```python
from build123d import *

# Parameters (mm, degrees)
SKETCH1_R           = 2.0701
BOSS_EXTRUDE1_DEPTH = 1.1684


with BuildPart() as part:
    # Sketch1 → Boss-Extrude1 (new body)
    with BuildSketch(Plane(origin=(0, 1.1684, 0), x_dir=(1, 0, 0), z_dir=(0, 1, 0))):
        with BuildLine():
            Line((16.856899662, 38.114124823), (13.80361258, 38.114124823))
            Line((13.80361258, 38.114124823), (-5.52378647, 18.786725773))
            Line((-5.52378647, 18.786725773), (-6.35, 16.792069862))
            Line((-6.35, 16.792069862), (-6.35, -10.541))
            Line((-6.35, -10.541), (-4.191, -12.7))
            Line((-4.191, -12.7), (4.191, -12.7))
            Line((4.191, -12.7), (6.35, -10.541))
            Line((6.35, -10.541), (6.35, 11.384871939))
            ThreePointArc((6.35, 11.384871939), (6.591682484, 12.599891837), (7.27993597, 13.62993597))
            Line((7.27993597, 13.62993597), (22.783868702, 29.133868702))
            Line((22.783868702, 29.133868702), (22.783868702, 32.187155783))
            Line((22.783868702, 32.187155783), (16.856899662, 38.114124823))
        make_face()
        with Locations((15.330256121, 30.660512242)):
            Circle(SKETCH1_R, mode=Mode.SUBTRACT)
        with Locations((0, 6.35)):
            Circle(SKETCH1_R, mode=Mode.SUBTRACT)
        with Locations((-2.085466914, 16.194084801)):
            Circle(SKETCH1_R, mode=Mode.SUBTRACT)
        with Locations((0, -6.35)):
            Circle(SKETCH1_R, mode=Mode.SUBTRACT)
        with Locations((6.35, 21.680256121)):
            Circle(SKETCH1_R, mode=Mode.SUBTRACT)
    extrude(amount=-BOSS_EXTRUDE1_DEPTH)


solid = part.part
```
Input: part model. Units: mm. Frame: model coordinates. A direction names the side the tool comes from. Coordinates: 2 decimals unless noted, no trailing zeros. Loops run counter-clockwise (first coordinate to the right, second up) from the corner with the lowest first, then second, coordinate; pieces in that order, holes last. Notation, with made-up numbers: M 14,-37 L 60,-37 A21 ccw 60,-10 Z; hole C 37.5,18 d4. An arc over 180 degrees is marked long. Use a Markdown table: item, result. Add a question column.
1) Draft query along X for faces 1 (the cylindrical face through (16.285, 0.592, -28.824)), 2 (the flat face through (5, 1.168, -13)), 3 (the flat face through (14.92, 0.59, -21.27)), 4 (the cylindrical face through (-0.97, 0.59, -17.94)). Return one class per face: +X half, -X half, draft (parallel to the pull), parting line (faces both ways), or undercut.
2) Section A-A, the plane z = 6.35. Return the cut outline in (x, y), plus the area to 3 significant figures.
3) Line query: L1, parallel to Z at x = 0.25, y = 0.65; L2, parallel to X at y = 0.8, z = -8.5; L3, parallel to Z at x = -1.75, y = 1. Output: solid intervals per line, ascending. Write a range as from..to.
4) Section C-C, the plane y = 0.25. Return the cut outline in (x, z) (3 decimals), plus the area to 3 significant figures.
5) Section D-D, the plane z = -24.5. Return the cut outline in (x, y), plus the area to 3 significant figures.
6) Section B-B, the plane x = 0.75. Return the cut outline in (y, z), plus the area to 3 significant figures.
7) Set-up query: faces 5 (the flat face through (6.35, 1, 0)), 6 (the cylindrical face through (-1.526, 0.592, 4.951)). Return all of +Z, -Z, +X, -X, +Y, -Y with unobstructed straight access to the full face (end or side cutting, diameter ignored); none if empty.
Answer below:
| question | item | result |
|---|---|---|
| 1 | face 1 | undercut |
| 1 | face 2 | draft |
| 1 | face 3 | +X half |
| 1 | face 4 | undercut |
| 2 | outline | M -6.35,0 L -2.07,0 L -2.07,1.17 L -6.35,1.17 Z; M 2.07,0 L 6.35,0 L 6.35,1.17 L 2.07,1.17 Z |
| 2 | area | 10.0 mm2 |
| 3 | L1 | -24.56..-8.4, -4.3..4.3, 8.4..12.7 |
| 3 | L2 | -6.35..6.35 |
| 3 | L3 | -22.56..-18.24, -14.15..-7.46, -5.24..5.24, 7.46..12.7 |
| 4 | outline | M -6.35,-16.792 L -5.524,-18.787 L 13.804,-38.114 L 16.857,-38.114 L 22.784,-32.187 L 22.784,-29.134 L 7.28,-13.63 A3.175 cw 6.35,-11.385 L 6.35,10.541 L 4.191,12.7 L -4.191,12.7 L -6.35,10.541 Z; hole C -2.085,-16.194 d4.14; hole C 0,-6.35 d4.14; hole C 0,6.35 d4.14; hole C 6.35,-21.68 d4.14; hole C 15.33,-30.661 d4.14 |
| 4 | area | 635 mm2 |
| 5 | outline | M 0.19,0 L 18.15,0 L 18.15,1.17 L 0.19,1.17 Z |
| 5 | area | 21.0 mm2 |
| 6 | outline | M 0,-25.06 L 1.17,-25.06 L 1.17,-8.28 L 0,-8.28 Z; M 0,-4.42 L 1.17,-4.42 L 1.17,4.42 L 0,4.42 Z; M 0,8.28 L 1.17,8.28 L 1.17,12.7 L 0,12.7 Z |
| 6 | area | 35.1 mm2 |
| 7 | face 5 | +Z, +X, +Y, -Y |
| 7 | face 6 | +Y, -Y |
